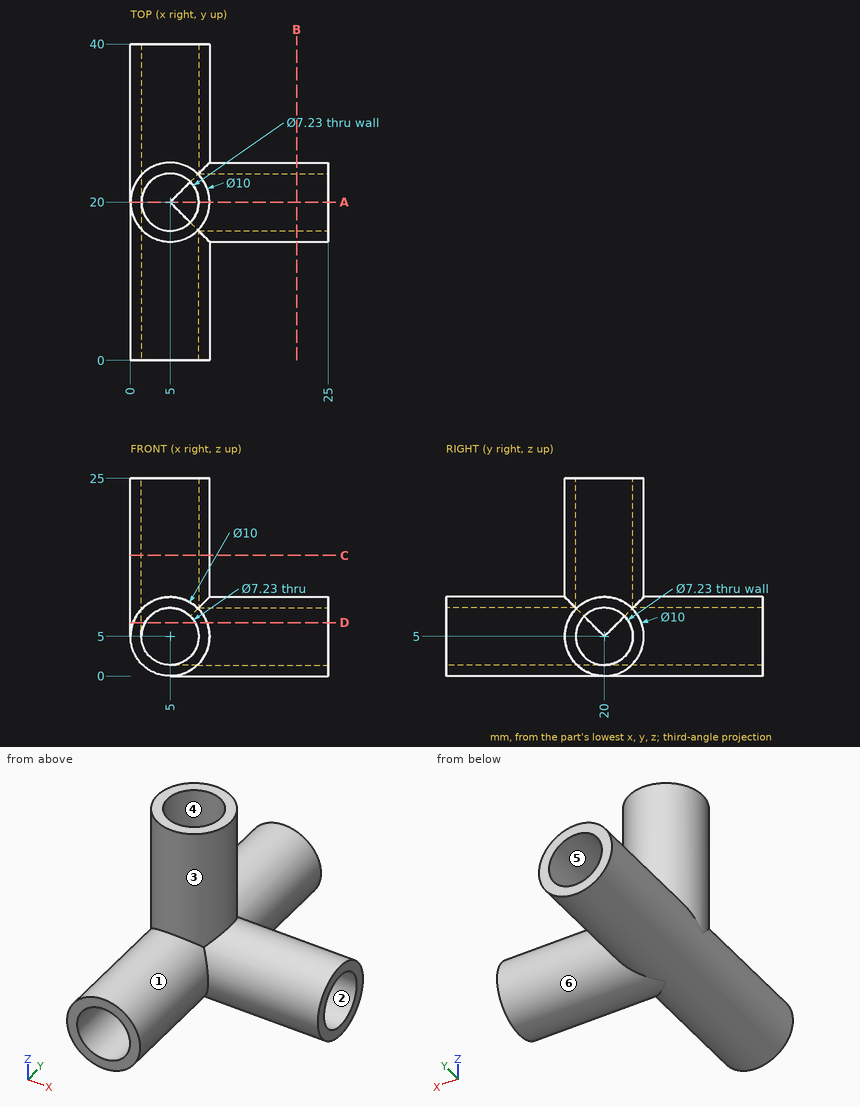
Here's the drawing with two shaded views (mm, measured from the low corner). I have some questions. A direction names the side the tool comes from. Coordinates: 2 decimals unless noted, no trailing zeros. Loops run counter-clockwise (first coordinate to the right, second up) from the corner with the lowest first, then second, coordinate; pieces in that order, holes last. Notation, with made-up numbers: M -33.75,32.5 L -26.75,32.5 A28 ccw -26.75,71.5 Z; hole C -3.5,35 d10. An arc over 180 degrees is marked long. Return JSON: item names as keys, results as strings. Group by question number.
Item 1: Imagine slicing it at C-C (z = 15.25). Please give me the cut outline in (x, y) (3 decimals), and give its area (3 significant figures).
Item 2: On a 3-axis mill with a long thin cutter (end or side, diameter ignored), from which of +Z, -Z, +X, -X, +Y, -Y can I reach the whole of each face in a straight line? I mean the marked faces 4, 5 and 6. Say none if no direction works.
Item 3: If I drill on L1, parallel to X at y = 13.5, z = 5 (3 decimals); L2, parallel to Y at x = 5, z = 21.25 (3 decimals); L3, parallel to Z at x = 21.25, y = 23, over which ranges is the centre line in solid material (lowest first)? Write a range as from..to.
Item 4: Imagine slicing it at D-D (z = 6.75). Please give me the cut outline in (x, y) (3 decimals).
Item 5: I'm going to push flat-ended pins straight in: pin 1 Ø12 at (x, y) = (19, 12.5) entering from +Z; pin 2 Ø2 at (x, y) = (5, 8) entering from +Z; pin 3 Ø3 at (y, z) = (22, 12) entering from +X. Where does each tip first touch, or does it pass through?
Item 6: Thinking about a two-plate mould opening in Y: for the marked faces 1, 2 and 3, which applies, released by +Y, released by -Y, zero draft, split by the parting line, or undercut?
Item 7: Imagine slicing it at B-B (x = 21). Please give me the cut outline in (y, z) (3 decimals), and give its area (3 significant figures).
Item 8: Imagine slicing it at A-A (y = 20). Please give me the cut outline in (x, z) (3 decimals).
Verdict:
{
 "1": {"outline": "C 5,20 d10; hole C 5,20 d7.23", "area": "37.5 mm^2"},
 "2": {"face 4": "+Z", "face 5": "+Y, -Y", "face 6": "+X"},
 "3": {"L1": "x = 0..1.385, 8.615..10", "L2": "y = 15..16.385, 23.615..25", "L3": "z = 1..2.98, 7.02..9"},
 "4": {"outline": "M 0.316,0 L 1.837,0 L 1.837,18.25 A3.615 cw 1.837,21.75 L 1.837,40 L 0.316,40 L 0.316,21.75 A5 ccw 0.316,18.25 Z; M 8.163,0 L 9.684,0 L 9.684,15.316 L 25,15.316 L 25,16.837 L 8.163,16.837 Z; M 8.163,23.163 L 25,23.163 L 25,24.684 L 9.684,24.684 L 9.684,40 L 8.163,40 Z"},
 "5": {"pin 1": "stops at z = 9.77", "pin 2": "stops at z = 10", "pin 3": "stops at x = 9.97"},
 "6": {"face 1": "zero draft", "face 2": "undercut", "face 3": "split by the parting line"},
 "7": {"outline": "C 20,5 d10; hole C 20,5 d7.23", "area": "37.5 mm^2"},
 "8": {"outline": "M 0,5 A5 ccw 5,0 L 25,0 L 25,1.385 L 5,1.385 A3.615 cw 1.385,5 L 1.385,25 L 0,25 Z; M 8.615,8.615 L 25,8.615 L 25,10 L 10,10 L 10,25 L 8.615,25 Z"}
}
